```python
from build123d import *

# Parameters (mm, degrees)
F1_DEPTH = 25
F3_DEPTH = 25
F4_R     = 2.8
F5_DEPTH = 2.801


with BuildPart() as f1:
    # F0 (on Front) → F1 (new body)
    with BuildSketch(Plane.XZ):
        Polygon((-12.5, 12.5), (-12.5, 0), (0, 0), (-2.8, 2.8), align=None)
        Polygon((2.8, 2.8), (0, 0), (12.5, 0), (12.5, 12.5), align=None)
        Polygon((-2.8, 2.8), (0, 0), (2.8, 2.8), align=None)
    extrude(amount=-F1_DEPTH)

    # F2 (on face) → F3 (join)
    with BuildSketch(Plane.YZ.offset(12.5)):
        Polygon((0, 0), (12.5, 0), (0, 12.5), align=None)
        Polygon((25, 12.5), (12.5, 0), (25, 0), align=None)
    extrude(amount=-F3_DEPTH)

    # F4 (on face) → F5 (cut, through all)
    with BuildSketch(Plane.XY.offset(2.8)):
        with Locations((0, 12.5)):
            Circle(F4_R)
    extrude(amount=-F5_DEPTH, mode=Mode.SUBTRACT)


solid = f1.part
```
Source: CAD feature listing. Evaluate the final solid. Frame: model axes, mm. A direction names the side the tool comes from. Give positions to 0.01 mm unless a question says otherwise; leave off trailing zeros. Loops run counter-clockwise (first coordinate to the right, second up) from the corner with the lowest first, then second, coordinate; pieces in that order, holes last. Notation, with made-up numbers: M -12,-3.5 L 22,-3.5 A30 cw 22,30.5 Z; hole C 8.25,24 d3. An arc over 180 degrees is marked long. Put each result on its own line as item: value.
Q1. Section B-B (x = 4). Return the cut outline in (y, z), and give its area (3 significant figures).
Response values:
outline: M 0,0 L 25,0 L 25,12.5 L 16.5,4 L 8.5,4 L 0,12.5 Z
area: 172 mm²
Q2. Line query: probe 1 along Y at (x, z) = (0, 0.75); probe 2 along X at (y, z) = (4.25, 10.75); probe 3 along Y at (x, z) = (3.25, 6). Output: solid intervals per line, ascending. Write a range as [from, to].
Response values:
probe 1: y = [0, 9.7], [15.3, 25]
probe 2: x = [-12.5, -10.75], [10.75, 12.5]
probe 3: y = [0, 6.5], [18.5, 25]
Q3. Pin query (flat end, axial travel): P1, Ø3, axis at x = -1, y = 11, coming from the +Z side; P2, Ø1.4, axis at x = 2, y = 10.5, coming from the +Z side. Return the tip coordinate at first contact, or that it passes through.
Response values:
P1: stops at z = 3
P2: stops at z = 2.8
Q4. Reachability of faces 1 (the flat face through (-12.5, 12, 6)), 2 (the flat face through (2, 10, 2.8)) from +Z, -Z, +X, -X, +Y, -Y: full face, straight path, thin tool, end or side. Return the list, or none.
Response values:
face 1: +Z, -Z, -X, +Y, -Y
face 2: +Z
Q5. Section C-C (y = 14.25). Return the cut outline in (x, z), and give its area (3 significant figures).
Response values:
outline: M -12.5,0 L -2.19,0 L -2.19,2.8 L -2.8,2.8 L -12.5,12.5 Z; M 2.19,0 L 12.5,0 L 12.5,12.5 L 2.8,2.8 L 2.19,2.8 Z
area: 152 mm²
Q6. Mould query, pull axis X, two halves, no side actions, for faces 3 (the flat face through (12.5, 12, 6)), 4 (the flat face through (0.2, 21.3, 8.8)), 5 (the flat face through (0, 0, 6)). Classes: released by +X, released by -X, zero draft, split by the parting line, or undercut.
Response values:
face 3: released by +X
face 4: undercut
face 5: zero draft
Q7. Section D-D (z = 7). Return the cut outline in (x, y), and give its area (3 significant figures).
Response values:
outline: M -12.5,0 L 12.5,0 L 12.5,25 L -12.5,25 Z; hole M -7,5.5 L 7,5.5 L 7,19.5 L -7,19.5 Z
area: 429 mm²
